from build123d import *
from OCP.BRepFilletAPI import BRepFilletAPI_MakeChamfer

# Parameters (mm, degrees)
SKETCH1_R           = 19.5
SKETCH1_R_2         = 17.1
BOSS_EXTRUDE1_DEPTH = 4.347826087
BOSS_EXTRUDE2_DEPTH = 1.08695652
CHAMFER1_SIZE       = 0.6
CHAMFER1_SIZE2      = 0.971
CUT_EXTRUDE1_DEPTH  = 29.687564735


with BuildPart() as part:
    # Sketch1 → Boss-Extrude1 (new body)
    with BuildSketch(Plane(origin=(0, 0, 0), x_dir=(1, 0, 0), z_dir=(0, 1, 0))):
        with Locations(Location((0, 0, 0), (0, 0, 270))):
            Circle(SKETCH1_R)
        with Locations(Location((0, 0, 0), (0, 0, 270))):
            Circle(SKETCH1_R_2, mode=Mode.SUBTRACT)
    extrude(amount=BOSS_EXTRUDE1_DEPTH)

    # Sketch2 → Boss-Extrude2 (add, symmetric)
    with BuildSketch(Plane.ZY.offset(19.5)):
        Polygon((0, 0.00928426), (-1.086956522, 2.173913043), (0, 4.338541827), (1.086956522, 2.173913043), align=None)
    extrude(amount=BOSS_EXTRUDE2_DEPTH, both=True)

    # Chamfer1: one chamfer whose edges measure the first distance from different faces: ONE call of the kernel's chamfer builder (chamfer() names one face for all edges)
    chamfer1_edges_1 = [part.edges().sort_by_distance(p)[0] for p in [
        (-20.58695652, 3.256227435, -0.543478261),
    ]]
    chamfer1_side_1 = [part.faces().sort_by_distance(p)[0] for p in [
        (-20.038389639, 3.251243161, -0.545981087),
    ]]
    chamfer1_edges_2 = [part.edges().sort_by_distance(p)[0] for p in [
        (-20.58695652, 1.091598652, -0.543478261),
    ]]
    chamfer1_side_2 = [part.faces().sort_by_distance(p)[0] for p in [
        (-20.038389639, 1.096582926, -0.545981087),
    ]]
    chamfer1_edges_3 = [part.edges().sort_by_distance(p)[0] for p in [
        (-20.58695652, 1.091598652, 0.543478261),
    ]]
    chamfer1_side_3 = [part.faces().sort_by_distance(p)[0] for p in [
        (-20.038389639, 1.096582926, 0.545981087),
    ]]
    chamfer1_edges_4 = [part.edges().sort_by_distance(p)[0] for p in [
        (-20.58695652, 3.256227435, 0.543478261),
    ]]
    chamfer1_side_4 = [part.faces().sort_by_distance(p)[0] for p in [
        (-20.038389639, 3.251243161, 0.545981087),
    ]]
    chamfer1 = BRepFilletAPI_MakeChamfer(part.part.solid().wrapped)
    for e in chamfer1_edges_1:
        chamfer1.Add(CHAMFER1_SIZE, CHAMFER1_SIZE2, e.wrapped, chamfer1_side_1[0].wrapped)  # the first distance lies on this face
    for e in chamfer1_edges_2:
        chamfer1.Add(CHAMFER1_SIZE, CHAMFER1_SIZE2, e.wrapped, chamfer1_side_2[0].wrapped)  # the first distance lies on this face
    for e in chamfer1_edges_3:
        chamfer1.Add(CHAMFER1_SIZE, CHAMFER1_SIZE2, e.wrapped, chamfer1_side_3[0].wrapped)  # the first distance lies on this face
    for e in chamfer1_edges_4:
        chamfer1.Add(CHAMFER1_SIZE, CHAMFER1_SIZE2, e.wrapped, chamfer1_side_4[0].wrapped)  # the first distance lies on this face
    add(Compound.cast(chamfer1.Shape()), mode=Mode.REPLACE)

    # Sketch3 → Cut-Extrude1 (cut, through all)
    with BuildSketch(Plane(origin=(0, 4.347826087, 0), x_dir=(1, 0, 0), z_dir=(0, 1, 0))):
        with BuildLine():
            Line((-17.274547751, 2.8), (-15.753094934, 2.8))
            ThreePointArc((-15.753094934, 2.8), (-16, 0), (-15.753094934, -2.8))
            Line((-15.753094934, -2.8), (-17.274547751, -2.8))
            ThreePointArc((-17.274547751, -2.8), (-17.5, 0), (-17.274547751, 2.8))
        make_face()
        with BuildLine():
            Line((11.062145006, 13.560197191), (10.301418598, 12.242580401))
            ThreePointArc((10.301418598, 12.242580401), (8, 13.856406461), (5.451676336, 15.042580401))
            Line((5.451676336, 15.042580401), (6.212402745, 16.360197191))
            ThreePointArc((6.212402745, 16.360197191), (8.75, 15.155444566), (11.062145006, 13.560197191))
        make_face()
        with BuildLine():
            Line((6.212402745, -16.360197191), (5.451676336, -15.042580401))
            ThreePointArc((5.451676336, -15.042580401), (8, -13.856406461), (10.301418598, -12.242580401))
            Line((10.301418598, -12.242580401), (11.062145006, -13.560197191))
            ThreePointArc((11.062145006, -13.560197191), (8.75, -15.155444566), (6.212402745, -16.360197191))
        make_face()
    extrude(amount=-CUT_EXTRUDE1_DEPTH, mode=Mode.SUBTRACT)


solid = part.part
The listing builds one solid part. Answer for the finished solid, in the listing's coordinates (mm). A direction names the side the tool comes from. Coordinates: 2 decimals unless noted, no trailing zeros. Write each loop counter-clockwise with the first axis right and the second up, starting at its lowest first coordinate (ties: lowest second). Pieces come first, ordered by that corner, then holes. Notation, with made-up numbers: M -23,66 L 26,66 A14 ccw 26,83 Z; hole C 64,-25.5 d8. An arc over 180 degrees is marked long. Use one line per item in the form item = value.
Item 1: Find section C-C, the plane z = -5.5. Give the vertices of the cut face in (x, y), plus the area to 3 significant figures.
Model answer:
outline = M -18.71,0 L -16.19,0 L -16.19,4.35 L -18.71,4.35 Z; M 16.19,0 L 18.71,0 L 18.71,4.35 L 16.19,4.35 Z
area = 21.9 mm2
Item 2: For faces 1 (the face through (-8.37, 2.14, -14.91)), 2 (the face through (17.4, 4.348, -0.1)), 3 (the face through (-19.732, 1.076, -0.536)), 4 (the face through (-20.158, 2.907, 0.41)), 5 (the face through (-19.732, 1.107, 0.551)), determine the directions among +Z, -Z, +X, -X, +Y, -Y from which every point of the face is accessible in a straight line to the end or side of a thin tool.
Model answer:
face_1 = +Y, -Y
face_2 = +Z, -Z, +X, -X, +Y
face_3 = -Z, -X, -Y
face_4 = +Z, -X, +Y
face_5 = +Z, -X, -Y
Item 3: Find section D-D, the plane y = 0.5. Give the vertices of the cut face in (x, z), plus the area to 3 significant figures.
Model answer:
outline = M -20.12,0 L -19.99,-0.25 L -19.5,-0.25 A19.5 ccw long -19.5,0.25 L -19.99,0.25 Z; hole M -17.27,-2.8 L -16.87,-2.8 A17.1 ccw 6.01,-16.01 L 6.21,-16.36 A17.5 ccw 11.06,-13.56 L 10.86,-13.21 A17.1 ccw 10.86,13.21 L 11.06,13.56 A17.5 ccw 6.21,16.36 L 6.01,16.01 A17.1 ccw -16.87,2.8 L -17.27,2.8 A17.5 ccw Z
area = 269 mm2
Item 4: Given P1, Ø2, axis at x = -12.5, y = 0.5, coming from the -Z side; P2, Ø1.5, axis at y = 2, z = 1.5, coming from the +X side; P3, Ø1, axis at x = -15.5, y = 2, coming from the -Z side, each flat-ended and moving along its own axis, determine where each tip first touches the part or whether it passes through.
Model answer:
P1 = -15.75
P2 = 19.49
P3 = -12.46
Item 5: Find section A-A, the plane x = 0. Give the vertices of the cut face in (y, z).
Model answer:
outline = M 0,-19.5 L 4.35,-19.5 L 4.35,-17.1 L 0,-17.1 Z; M 0,17.1 L 4.35,17.1 L 4.35,19.5 L 0,19.5 Z
Item 6: Find the intervals of material crossed by probe 1 along Z at (x, y) = (5, 2.9); probe 2 along Z at (x, y) = (9, 2.55); probe 3 along X at (y, z) = (4, 13), in increasing order.
Model answer:
probe_1 = -18.85 to -16.35, 16.35 to 18.85
probe_2 = -17.3 to -15.01, 15.01 to 17.3
probe_3 = -14.53 to -11.11, 11.11 to 14.53
Item 7: Find section B-B, the plane y = 3. Give the vertices of the cut face in (x, z).
Model answer:
outline = M -20.36,0 L -19.99,-0.67 L -19.49,-0.67 A19.5 ccw long -19.49,0.67 L -19.99,0.67 Z; hole M -17.27,-2.8 L -16.87,-2.8 A17.1 ccw 6.01,-16.01 L 6.21,-16.36 A17.5 ccw 11.06,-13.56 L 10.86,-13.21 A17.1 ccw 10.86,13.21 L 11.06,13.56 A17.5 ccw 6.21,16.36 L 6.01,16.01 A17.1 ccw -16.87,2.8 L -17.27,2.8 A17.5 ccw Z
Item 8: The mould has two halves that part along Z. Classify faces 6 (the face through (-19.732, 3.271, 0.536)), 7 (the face through (-19.73, 3.24, -0.55)), 8 (the face through (-8.732, 2.143, 14.702)), 9 (the face through (17.1, 2.1, 0.2)): released by +Z, released by -Z, zero draft, split by the parting line, or undercut.
Model answer:
face_6 = released by +Z
face_7 = released by -Z
face_8 = undercut
face_9 = undercut
